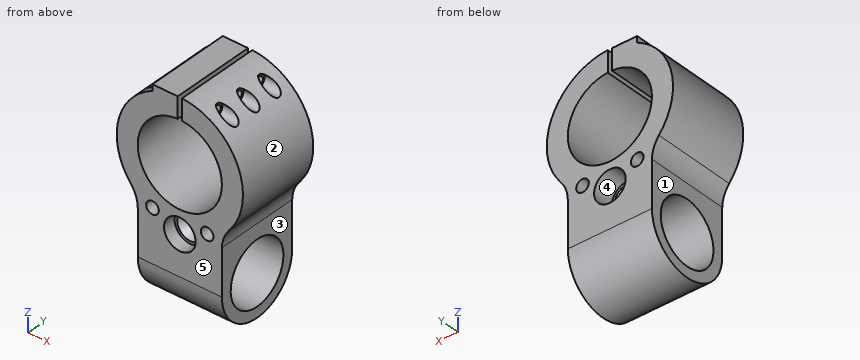
```python
from build123d import *

# Parameters (mm, degrees)
SKETCH1_R                                    = 30
SKETCH1_R_2                                  = 20
BOSS_EXTRUDE1_DEPTH                          = 40
SKETCH2_W                                    = 2
SKETCH2_H                                    = 30
CUT_EXTRUDE1_DEPTH                           = 59.309518948
BOSS_EXTRUDE2_START                          = -40
BOSS_EXTRUDE2_DEPTH                          = 40
CBORE_FOR_M4_HEX_SOCKET_HEAD_CAP_SCR_2_COUNT = 2
CBORE_FOR_M4_HEX_SOCKET_HEAD_CAP_SCR_2_PITCH = 12
CBORE_FOR_M4_HEX_SOCKET_HEAD_CAP_SCR_3_COUNT = 2
CBORE_FOR_M4_HEX_SOCKET_HEAD_CAP_SCR_3_PITCH = 24
SKETCH6_R                                    = 3.75
CUT_EXTRUDE2_DEPTH                           = 66.946948375
F_5_4_5_4_DIAMETER_HOLE1_D                   = 4.2
SKETCH10_R                                   = 3
CUT_EXTRUDE3_DEPTH                           = 11
BOSS_EXTRUDE4_START                          = -20
BOSS_EXTRUDE4_OUTLINE_R                      = 15
BOSS_EXTRUDE4_DEPTH                          = 40
FILLET1_R                                    = 15
SKETCH22_R                                   = 3.25
CUT_EXTRUDE4_DEPTH                           = 87.023252752
SKETCH23_R                                   = 7.5
CUT_EXTRUDE5_DEPTH                           = 10
CHAMFER1_SIZE                                = 3
CUT_EXTRUDE6_START                           = -6
SKETCH24_R                                   = 7.5
CUT_EXTRUDE6_DEPTH                           = 6
CHAMFER2_SIZE                                = 3
F_6_0MM_DOWEL_HOLE1_D                        = 6


# Read off the part's stored shape, not the designer's step: Boss-Extrude4
with BuildPart() as part:
    # Sketch1 → Boss-Extrude1 (new body)
    with BuildSketch(Plane(origin=(0, 0, 0), x_dir=(1, 0, 0), z_dir=(0, 1, 0))):
        with Locations(Location((0, 0, 0), (0, 0, 270))):
            Circle(SKETCH1_R)
        with Locations(Location((0, 0, 0), (0, 0, 270))):
            Circle(SKETCH1_R_2, mode=Mode.SUBTRACT)
    extrude(amount=BOSS_EXTRUDE1_DEPTH)

    # Sketch2 → Cut-Extrude1 (cut, through all)
    with BuildSketch(Plane(origin=(0, 40, 0), x_dir=(1, 0, 0), z_dir=(0, 1, 0))):
        with Locations((0, -15)):
            Rectangle(SKETCH2_W, SKETCH2_H)
    extrude(amount=-CUT_EXTRUDE1_DEPTH, mode=Mode.SUBTRACT)

    # Sketch3 → Boss-Extrude2 (add)
    with BuildSketch(Plane(origin=(0, 40, 0), x_dir=(1, 0, 0), z_dir=(0, 1, 0)).offset(BOSS_EXTRUDE2_START)):
        with BuildLine():
            Line((-1, -29.983328701), (-13, -29.983328701))
            Line((-13, -29.983328701), (-13, -27.037011669))
            ThreePointArc((-13, -27.037011669), (-7.153334608, -29.134683866), (-1, -29.983328701))
        make_face()
    extrude(amount=BOSS_EXTRUDE2_DEPTH)

    # Sketch5 → CBORE for M4 Hex Socket Head Cap Screw1 (revolve, cut)
    with BuildSketch(Plane(origin=(-13, 32, 24.979156528), x_dir=(0, 0, 1), z_dir=(0, 1, 0))):
        Polygon((0, 0), (0, 13.351936393), (2.25, 12), (2.25, 4), (3.75, 4), (3.75, 0), align=None)
    cbore_for_m4_hex_socket_head_cap_screw1 = revolve(axis=Axis((-19.35, 32, 24.979156528), (1, 0, 0)), mode=Mode.SUBTRACT)

    # CBORE for M4 Hex Socket Head Cap Scr 2: CBORE for M4 Hex Socket Head Cap Screw1 ×2
    with Locations(*[(0, -i * CBORE_FOR_M4_HEX_SOCKET_HEAD_CAP_SCR_2_PITCH, 0) for i in range(1, CBORE_FOR_M4_HEX_SOCKET_HEAD_CAP_SCR_2_COUNT)]):
        add(cbore_for_m4_hex_socket_head_cap_screw1, mode=Mode.SUBTRACT)

    # CBORE for M4 Hex Socket Head Cap Scr 3: CBORE for M4 Hex Socket Head Cap Screw1 ×2
    with Locations(*[(0, -i * CBORE_FOR_M4_HEX_SOCKET_HEAD_CAP_SCR_3_PITCH, 0) for i in range(1, CBORE_FOR_M4_HEX_SOCKET_HEAD_CAP_SCR_3_COUNT)]):
        add(cbore_for_m4_hex_socket_head_cap_screw1, mode=Mode.SUBTRACT)

    # Sketch6 → Cut-Extrude2 (cut, through all)
    with BuildSketch(Plane.ZY.offset(13)):
        with Locations((24.979156528, 32)):
            Circle(SKETCH6_R)
        with Locations((24.979156528, 20)):
            Circle(SKETCH6_R)
        with Locations((24.979156528, 8)):
            Circle(SKETCH6_R)
    extrude(amount=CUT_EXTRUDE2_DEPTH, mode=Mode.SUBTRACT)

    # Ø5.4 (5.4) Diameter Hole1 (through all)
    with Locations(Plane.ZY.offset(-1)):
        with Locations((24.979156528, 8), (24.979156528, 20), (24.979156528, 32)):
            Hole(F_5_4_5_4_DIAMETER_HOLE1_D / 2)

    # Sketch10 → Cut-Extrude3 (cut)
    with BuildSketch(Plane.ZY.offset(-22)):
        with Locations((24.979156528, 8)):
            Circle(SKETCH10_R)
        with Locations((24.979156528, 32)):
            Circle(SKETCH10_R)
        with Locations((24.979156528, 20)):
            Circle(SKETCH10_R)
    extrude(amount=CUT_EXTRUDE3_DEPTH, mode=Mode.SUBTRACT)

    # Boss-Extrude4 outline → Boss-Extrude4 (add)
    with BuildSketch(Plane(origin=(0, 0, 0), x_dir=(0, 0, -1), z_dir=(1, 0, 0)).offset(BOSS_EXTRUDE4_START)):
        with BuildLine():
            ThreePointArc((50, 0), (70, 20), (50, 40))
            Line((50, 40), (28, 40))
            Line((28, 40), (28, 0))
            Line((28, 0), (50, 0))
        make_face()
        with Locations((50, 20)):
            Circle(BOSS_EXTRUDE4_OUTLINE_R, mode=Mode.SUBTRACT)
    extrude(amount=BOSS_EXTRUDE4_DEPTH)

    # Fillet1
    # the kernel refuses this fillet: 15 mm, written as the material it adds along each edge
    with BuildSketch(Plane(origin=(10.770329614, 40, -28), x_dir=(0.8085477056225361, 0, 0.5884306311983875), z_dir=(0, -1, 0))) as fillet1_piece_1:
        with BuildLine():
            CenterArc((19.419330938, -14.488463805), FILLET1_R, 105.006250165, 37.84908673)
            Line((7.462628814, -5.431020771), (0, 0))
            ThreePointArc((0, 0), (7.767732375, -1.023072389), (15.53546475, 0))
        make_face()
    extrude(amount=40)
    with BuildSketch(Plane(origin=(-10.770329614, 40, -28), x_dir=(-0.8085477056225359, 0, 0.5884306311983878), z_dir=(0, -1, 0))) as fillet1_piece_2:
        with BuildLine():
            CenterArc((19.419330938, 14.488463805), FILLET1_R, 217.144663105, 37.84908673)
            Line((7.462628814, 5.431020771), (0, 0))
            ThreePointArc((0, 0), (7.767732375, 1.023072389), (15.53546475, 0))
        make_face()
    extrude(amount=40)

    # Sketch22 → Cut-Extrude4 (cut, through all)
    with BuildSketch(Plane(origin=(0, 40, 0), x_dir=(1, 0, 0), z_dir=(0, 1, 0))):
        with Locations(Location((0, 31, 0), (0, 0, 270))):
            Circle(SKETCH22_R)
    extrude(amount=-CUT_EXTRUDE4_DEPTH, mode=Mode.SUBTRACT)

    # Sketch23 → Cut-Extrude5 (cut)
    with BuildSketch(Plane(origin=(0, 40, 0), x_dir=(1, 0, 0), z_dir=(0, 1, 0))):
        with Locations(Location((0, 31, 0), (0, 0, 270))):
            Circle(SKETCH23_R)
    extrude(amount=-CUT_EXTRUDE5_DEPTH, mode=Mode.SUBTRACT)

    # Chamfer1
    chamfer1_edges = [part.edges().sort_by_distance(p)[0] for p in [
        (0, 30, -34.25),
    ]]
    chamfer(chamfer1_edges, length=CHAMFER1_SIZE)

    # Sketch24 → Cut-Extrude6 (cut)
    with BuildSketch(Plane.XZ.offset(CUT_EXTRUDE6_START)):
        with Locations(Location((0, -31, 0), (0, 0, 90))):
            Circle(SKETCH24_R)
    extrude(amount=CUT_EXTRUDE6_DEPTH, mode=Mode.SUBTRACT)

    # Chamfer2
    chamfer2_edges = [part.edges().sort_by_distance(p)[0] for p in [
        (0, 6, -34.25),
    ]]
    chamfer(chamfer2_edges, length=CHAMFER2_SIZE)

    # Ø6.0mm Dowel Hole1 (through all)
    with Locations(Plane(origin=(0, 0, 0), x_dir=(-1, 0, 0), z_dir=(0, -1, 0))):
        with Locations((13, 25), (-13, 25)):
            Hole(F_6_0MM_DOWEL_HOLE1_D / 2)


solid = part.part
```
Can you work these out from the model? Positions are in its coordinate system, mm. Face numbers are marked on the shaded views. A direction names the side the tool comes from. Coordinates: 2 decimals unless noted, no trailing zeros. Loops run counter-clockwise (first coordinate to the right, second up) from the corner with the lowest first, then second, coordinate; pieces in that order, holes last. Notation, with made-up numbers: M 42.5,51 L 76.5,51 A20 ccw 76.5,71 Z; hole C 76,-22.5 d6. An arc over 180 degrees is marked long. Put each result on its own line as item: value. Start each with the question number.
(1) Imagine slicing it at B-B on y = 3. List the corners of the cut face in (x, z) for me.
(2) We'd pull the mould along X, two halves only. Please class the marked faces 3, 4 and 5: +X half, -X half, draft (parallel to the pull), parting line (faces both ways), or undercut.
(3) Will these pins go through, and if not, where does the flat tip stop? pin 1 Ø1.5 at (x, y) = (-3, 19) entering from -Z; pin 2 Ø10 at (y, z) = (8, 24.98) entering from +X; pin 3 Ø3 at (y, z) = (7, 24.5) entering from +X; pin 4 Ø3.5 at (y, z) = (20, 24.98) entering from +X (3 decimals).
(4) Which directions (+Z, -Z, +X, -X, +Y, -Y) give clear straight access to the entire face, cutting with the end or side of a thin tool? Please do the marked faces 1 and 2.
(5) Imagine slicing it at D-D on z = -4. List the corners of the cut face in (x, y) for me, and give its area (3 significant figures).
(6) Imagine slicing it at C-C on z = -47. List the corners of the cut face in (x, y) for me, and give its area (3 significant figures).
(7) I need wall thicknesses on probe 1 along Y at (x, z) = (3, -50); probe 2 along Z at (x, y) = (3, 24); probe 3 along Z at (x, y) = (-11, 15). Which ranges of each line are inside material? Lowest first, please.
(8) Imagine slicing it at A-A on z = -31. List the corners of the cut face in (x, y) for me, and give its area (3 significant figures).
Worked answers:
1. outline: M -23.33,-18.86 A15 cw -20,-28 L -20,-60.54 L 20,-60.54 L 20,-28 A15 cw 23.33,-18.86 A30 ccw 1,29.98 L 1,19.97 A20 cw long -1,19.97 L -1,29.98 L -13,29.98 L -13,27.04 A30 ccw Z; hole C -13,-25 d6; hole C 0,-31 d15; hole C 13,-25 d6
2. face 3: +X half
2. face 4: undercut
2. face 5: draft
3. pin 1: stops at z = -70
3. pin 2: stops at x = 22.38
3. pin 3: stops at x = 11
3. pin 4: passes through
4. face 1: -Z, -X, +Y, -Y
4. face 2: +X, +Y, -Y
5. outline: M -29.73,0 L -19.6,0 L -19.6,40 L -29.73,40 Z; M 19.6,0 L 29.73,0 L 29.73,40 L 19.6,40 Z
5. area: 811 mm2
6. outline: M -20,0 L 20,0 L 20,5.3 L -20,5.3 Z; M -20,34.7 L 20,34.7 L 20,40 L -20,40 Z
6. area: 424 mm2
7. probe 1: y = 0 to 5, 35 to 40
7. probe 2: z = -69.6 to -64.46, -35.54 to -32.25, -29.75 to -19.77, 19.77 to 29.85
7. probe 3: z = -69.36 to -64.14, -35.86 to -27.24, -22.76 to -16.7, 16.7 to 29.98
8. outline: M -20,0 L -7.5,0 L -7.5,6 L -6.25,6 L -3.25,9 L -3.25,27 L -6.25,30 L -7.5,30 L -7.5,40 L -20,40 Z; M 3.25,9 L 6.25,6 L 7.5,6 L 7.5,0 L 20,0 L 20,40 L 7.5,40 L 7.5,30 L 6.25,30 L 3.25,27 Z
8. area: 1,190 mm2
